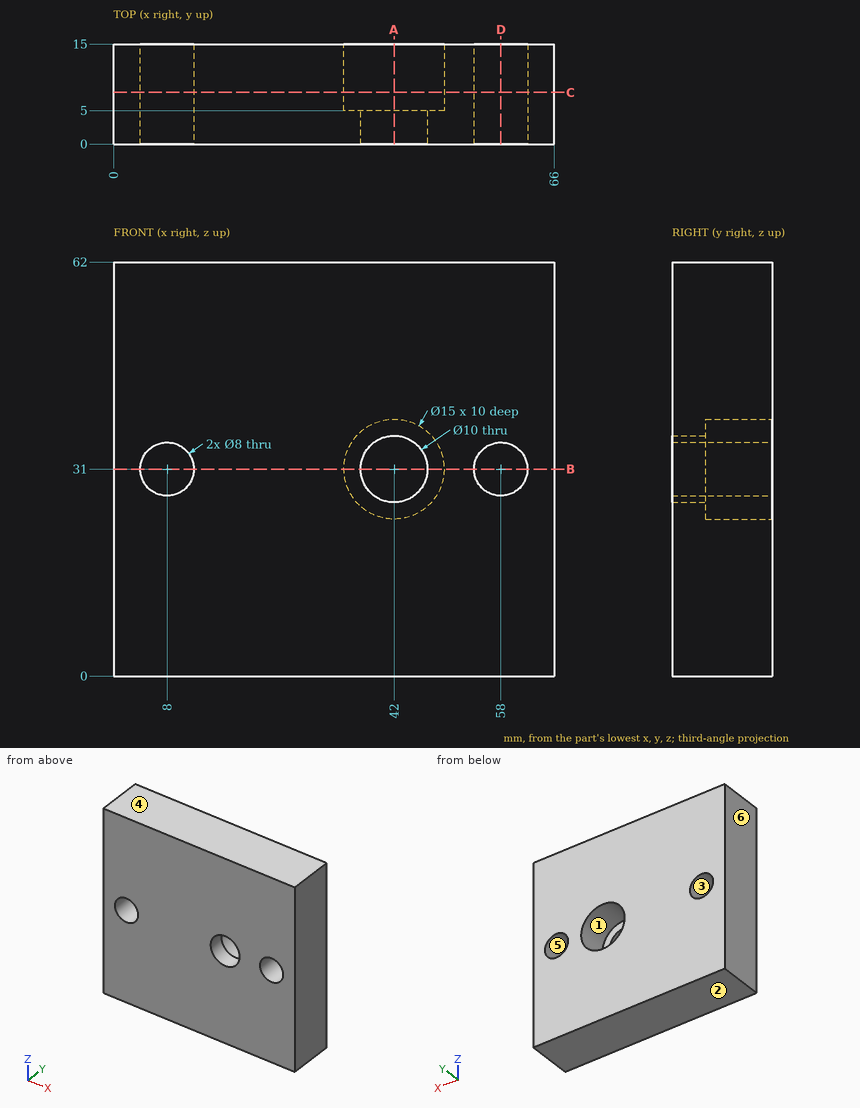
Can you work these out from the drawing? Everything is in mm from the part's minimum corner. A direction names the side the tool comes from. Coordinates: 2 decimals unless noted, no trailing zeros. Loops run counter-clockwise (first coordinate to the right, second up) from the corner with the lowest first, then second, coordinate; pieces in that order, holes last. Notation, with made-up numbers: (74, 53.5) - (85, 53.5) arc R12 ccw to (85, 62.5) - close; hole circle Ø4 at (35.5, 63). An arc over 180 degrees is marked (long way). Answer as CSV lines item,"result".
Q1. If we section it at B-B, the plane z = 31: Write out the boundary of the cut face in (x, y).
Response:
outline,"(0, 0) - (4, 0) - (4, 15) - (0, 15) - close; (12, 0) - (37, 0) - (37, 5) - (34.5, 5) - (34.5, 15) - (12, 15) - close; (47, 0) - (54, 0) - (54, 15) - (49.5, 15) - (49.5, 5) - (47, 5) - close; (62, 0) - (66, 0) - (66, 15) - (62, 15) - close"
Q2. For the marked faces 1 and 2, which set-ups out of +Z, -Z, +X, -X, +Y, -Y let a thin tool reach every point of the face, with its end or its side?
Response:
face 1,"+Y"
face 2,"-Z, +X, -X, +Y, -Y"
Q3. If we section it at D-D, the plane x = 58: Write out the boundary of the cut face in (y, z), and give its area (3 significant figures).
Response:
outline,"(0, 0) - (15, 0) - (15, 27) - (0, 27) - close; (0, 35) - (15, 35) - (15, 62) - (0, 62) - close"
area,"810 mm2"
Q4. If I drill on L1, parallel to X at y = 9, z = 31; L2, parallel to X at y = 4.75, z = 31; L3, parallel to Z at x = 42, y = 5.5, over which ranges is the centre line in solid material (lowest first)? Write a range as [from, to].
Response:
L1,"[0, 4], [12, 34.5], [49.5, 54], [62, 66]"
L2,"[0, 4], [12, 37], [47, 54], [62, 66]"
L3,"[0, 23.5], [38.5, 62]"
Q5. If we section it at A-A, the plane x = 42: Write out the boundary of the cut face in (y, z), and give its area (3 significant figures).
Response:
outline,"(0, 0) - (15, 0) - (15, 23.5) - (5, 23.5) - (5, 26) - (0, 26) - close; (0, 36) - (5, 36) - (5, 38.5) - (15, 38.5) - (15, 62) - (0, 62) - close"
area,"730 mm2"
Q6. We'd pull the mould along Z, two halves only. Please class the marked faces 3, 4, 5 and 6: pulls with the +Z half, pulls with the -Z half, needs draft (parallel to the pull), parting line crosses it, or undercut.
Response:
face 3,"undercut"
face 4,"pulls with the +Z half"
face 5,"undercut"
face 6,"needs draft"
Q7. If we section it at C-C, the plane y = 7.75: Write out the boundary of the cut face in (x, z), and give its area (3 significant figures).
Response:
outline,"(0, 0) - (66, 0) - (66, 62) - (0, 62) - close; hole circle Ø8 at (8, 31); hole circle Ø15 at (42, 31); hole circle Ø8 at (58, 31)"
area,"3,810 mm2"
Q8. For pin 1 (7.5 mm diameter, centred on x = 45, z = 28, fed in from +Y), with a flat end and sliding along its axis, tell me the tip position at first contact or that it passes through.
Response:
pin 1,"y = 15"
